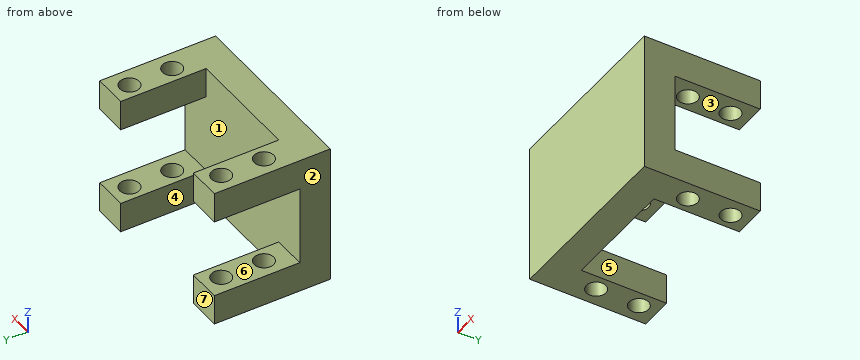
```python
from build123d import *

# Parameters (mm, degrees)
EXTRUDE_1_DEPTH     = 23
HOLE_WIZARD_1_D     = 3.2
SKETCH_4_W          = 13
SKETCH_4_H          = 14
CUT_EXTRUDE_1_DEPTH = 39.977557645


with BuildPart() as part:
    # 草图1 → 凸台-拉伸1 (new body)
    with BuildSketch(Plane.XY):
        Polygon((-15, -9.5), (15, -9.5), (15, 9.5), (9.5, 9.5), (9.5, -4.5), (-9.5, -4.5), (-9.5, 9.5), (-15, 9.5), align=None)
    extrude(amount=EXTRUDE_1_DEPTH)

    # 孔1 (through all)
    with Locations(Plane(origin=(0, 0, 0), x_dir=(-1, 0, 0), z_dir=(0, 0, -1))):
        with Locations((12, 6.5), (12, -0.5), (-12, -0.5), (-12, 6.5)):
            Hole(HOLE_WIZARD_1_D / 2)

    # 草图4 → 切除-拉伸1 (cut, through all)
    with BuildSketch(Plane(origin=(15, 0, 0), x_dir=(0, 0, -1), z_dir=(1, 0, 0))):
        with Locations((-11.5, 2.5)):
            Rectangle(SKETCH_4_W, SKETCH_4_H)
    extrude(amount=-CUT_EXTRUDE_1_DEPTH, mode=Mode.SUBTRACT)


solid = part.part
```
Geometry: final body of the model. Coordinates: model frame, mm. Face numbers are marked on the shaded views. A direction names the side the tool comes from. Coordinates: 2 decimals unless noted, no trailing zeros. Order: outer loops, then holes, each group sorted by start corner. A loop starts at its lowest first (then second) coordinate and runs counter-clockwise, first axis right, second up.
Item 1: Section query B-B (z = 2.25). Output: boundary loops of the cut face in (x, y).
Answer:
outline: (-15, -9.5) - (15, -9.5) - (15, 9.5) - (9.5, 9.5) - (9.5, -4.5) - (-9.5, -4.5) - (-9.5, 9.5) - (-15, 9.5) - close; hole circle Ø3.2 at (-12, -0.5); hole circle Ø3.2 at (-12, 6.5); hole circle Ø3.2 at (12, -0.5); hole circle Ø3.2 at (12, 6.5)
Item 2: Section query D-D (y = 2.25). Output: boundary loops of the cut face in (x, z).
Answer:
outline: (-15, 0) - (-9.5, 0) - (-9.5, 5) - (-15, 5) - close; (-15, 18) - (-9.5, 18) - (-9.5, 23) - (-15, 23) - close; (9.5, 0) - (15, 0) - (15, 5) - (9.5, 5) - close; (9.5, 18) - (15, 18) - (15, 23) - (9.5, 23) - close
Item 3: Section query A-A (y = 6.5). State how many separate pieces and enclosed holes the cut face has, then the cut area to 3 significant figures.
Answer:
separate pieces: 8
enclosed holes: 0
area: 46.0 mm2
Item 4: Draft query along X for the marked faces 1, 2, 3 and 4. Return one class per face: released by +X, released by -X, zero draft, split by the parting line, or undercut.
Answer:
face 1: undercut
face 2: released by -X
face 3: zero draft
face 4: undercut
Item 5: Material intervals for line 1 along Y through (x, z) = (-12, 1.9); line 2 along X through (y, z) = (7.5, 19); line 3 along X through (y, z) = (-2.25, 21.25), sorted ascending.
Answer:
line 1: y = -9.5 to -2.1, 1.1 to 4.9, 8.1 to 9.5
line 2: x = -15 to -13.25, -10.75 to -9.5, 9.5 to 10.75, 13.25 to 15
line 3: x = -15 to -9.5, 9.5 to 15
Item 6: Section query C-C (x = -12). Output: boundary loops of the cut face in (y, z), then the cut area to 3 significant figures.
Answer:
outline: (-9.5, 0) - (-2.1, 0) - (-2.1, 5) - (-4.5, 5) - (-4.5, 18) - (-2.1, 18) - (-2.1, 23) - (-9.5, 23) - close; (1.1, 0) - (4.9, 0) - (4.9, 5) - (1.1, 5) - close; (1.1, 18) - (4.9, 18) - (4.9, 23) - (1.1, 23) - close; (8.1, 0) - (9.5, 0) - (9.5, 5) - (8.1, 5) - close; (8.1, 18) - (9.5, 18) - (9.5, 23) - (8.1, 23) - close
area: 191 mm2
Item 7: Access query for the marked faces 5, 6 and 7. Directions: +Z, -Z, +X, -X, +Y, -Y. A direction counts if a zero-diameter tool reaches every point of the face in a straight line with its end or side. Return the directions, or none.
Answer:
face 5: +Z, -Z, +Y
face 6: +X, -X, +Y
face 7: +Z, -Z, +X, -X, +Y
Item 8: Contact query for flat-ended pins moving along their axis: P1, Ø10, axis at x = 2, z = 16.5, coming from the +Y side; P2, Ø1.9, axis at x = 12, y = 6.5, coming from the -Z side. Output: stop coordinate, or through.
Answer:
P1: stops at y = -4.5
P2: passes through
